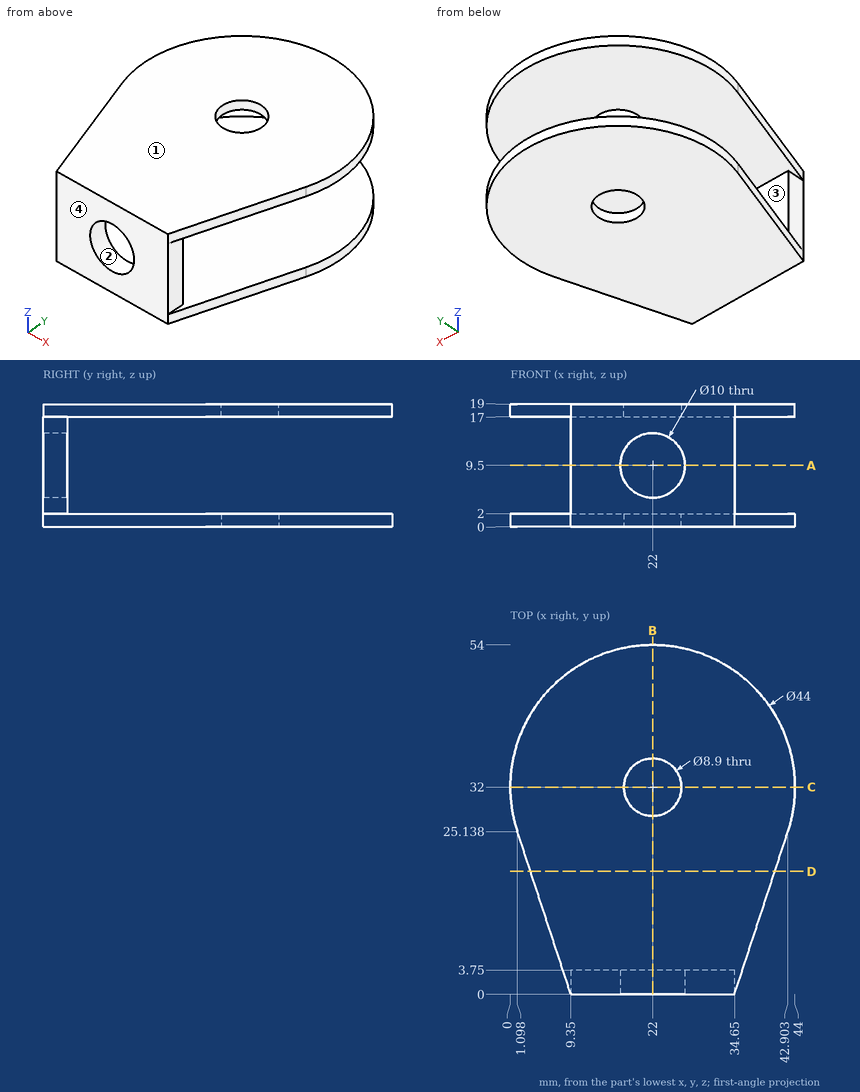
Here's the drawing with two shaded views (mm, measured from the low corner). I have some questions. A direction names the side the tool comes from. Give positions to 0.01 mm unless a question says otherwise; leave off trailing zeros. Order: outer loops, then holes, each group sorted by start corner. A loop starts at its lowest first (then second) coordinate and runs counter-clockwise, first axis right, second up.
Q1. For the marked faces 3 and 4, which set-ups out of +Z, -Z, +X, -X, +Y, -Y let a thin tool reach every point of the face, with its end or its side?
Q2. I'm going to push flat-ended pins straight in: P1, Ø1.1, axis at y = 1, z = 8, coming from the +X side; P2, Ø8, axis at y = 11.5, z = 4.5, coming from the -X side; P3, Ø1, axis at x = 17.5, z = 13.5, coming from the +Y side. Where does each tip first touch, or does it pass through?
Q3. We'd pull the mould along X, two halves only. Please class the marked faces 1 and 2: +X half, -X half, draft (parallel to the pull), parting line (faces both ways), or undercut.
Q4. Suppose I cut it at B-B, the plane x = 22. Write out the boundary of the cut face in (y, z), and give its area (3 significant figures).
Q5. Suppose I cut it at A-A, the plane z = 9.5. Write out the boundary of the cut face in (x, y).
Q6. Suppose I cut it at C-C, the plane y = 32. Write out the boundary of the cut face in (x, z).
Q7. If I drill on line 1 along Z through (x, y) = (32, 16.5); line 2 along X through (y, z) = (32, 0.9); line 3 along Y through (x, z) = (22, 18.4), over which ranges is the centre line in solid material (lowest first)?
Q8. Suppose I cut it at D-D, the plane y = 19. Write out the boundary of the cut face in (x, z).
Solution:
1. face 3: +X, -X, +Y
1. face 4: +Z, -Z, +X, -X, -Y
2. P1: stops at x = 34.65
2. P2: stops at x = 4.55
2. P3: stops at y = 3.75
3. face 1: draft
3. face 2: undercut
4. outline: (0, 0) - (27.55, 0) - (27.55, 2) - (3.75, 2) - (3.75, 4.5) - (0, 4.5) - close; (0, 14.5) - (3.75, 14.5) - (3.75, 17) - (27.55, 17) - (27.55, 19) - (0, 19) - close; (36.45, 0) - (54, 0) - (54, 2) - (36.45, 2) - close; (36.45, 17) - (54, 17) - (54, 19) - (36.45, 19) - close
4. area: 199 mm2
5. outline: (9.35, 0) - (17, 0) - (17, 3.75) - (9.35, 3.75) - close; (27, 0) - (34.65, 0) - (34.65, 3.75) - (27, 3.75) - close
6. outline: (0, 0) - (17.55, 0) - (17.55, 2) - (0, 2) - close; (0, 17) - (17.55, 17) - (17.55, 19) - (0, 19) - close; (26.45, 0) - (44, 0) - (44, 2) - (26.45, 2) - close; (26.45, 17) - (44, 17) - (44, 19) - (26.45, 19) - close
7. line 1: z = 0 to 2, 17 to 19
7. line 2: x = 0 to 17.55, 26.45 to 44
7. line 3: y = 0 to 27.55, 36.45 to 54
8. outline: (3.11, 0) - (40.89, 0) - (40.89, 2) - (3.11, 2) - close; (3.11, 17) - (40.89, 17) - (40.89, 19) - (3.11, 19) - close
